Could you check a few things on this model? Use its own coordinates, in mm. Give positions to 0.01 mm unless a question says otherwise; leave off trailing zeros. Answer in a Markdown table with one row per item.
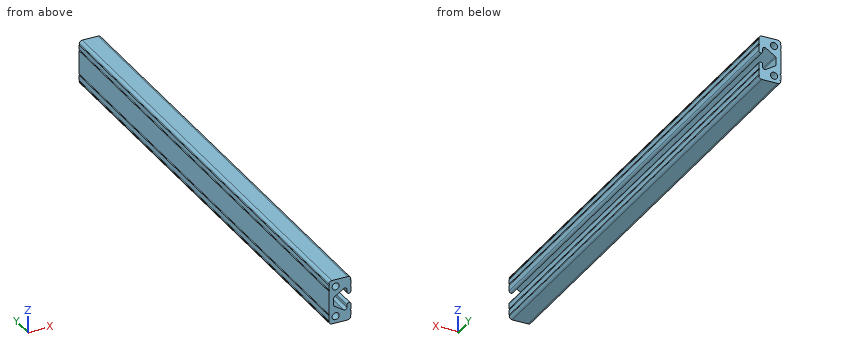
Solid Edge part; units mm, degrees
sketch "Sketch1" plane through (0, 0, 0) normal (0, 0, 1) x (1, 0, 0)
  line L0 (0, 0) -> (0, 279.4)
sketch "Sketch2" plane through (0, 0, 0) normal (0, -1, 0) x (1, 0, 0)
  line L0 (4.572, 12.7) -> (-4.572, 12.7)
  arc A0 (-4.572, 12.7) -> (-6.35, 10.922) centre (-4.572, 10.922) ccw
  line L1 (-6.35, 10.922) -> (-6.35, -10.922)
  arc A1 (-4.572, -12.7) -> (-6.35, -10.922) centre (-4.572, -10.922) cw
  line L2 (-4.572, -12.7) -> (4.572, -12.7)
  arc A2 (4.572, -12.7) -> (6.35, -10.922) centre (4.572, -10.922) ccw
  line L3 (6.35, -10.922) -> (6.35, 10.922)
  arc A3 (6.35, 10.922) -> (4.572, 12.7) centre (4.572, 10.922) ccw
sweep "SweptProtrusion1" add profiles "Sketch2" path "Sketch1"
sketch "Sketch3" plane through (0, 0, 0) normal (0, 0, 1) x (1, 0, 0)
  line L0 (0, 0) -> (0, 279.4)
sketch "Sketch4" plane through (-6.35, 0, 6.35) normal (0, -1, 0) x (1, 0, 0)
  circle A0 centre (3.9624, 2.3876) radius 2.032
sweep "SweptCutout1" cut profiles "Sketch4" path "Sketch3"
sketch "Sketch5" plane through (0, 0, 0) normal (0, 0, 1) x (1, 0, 0)
  line L0 (0, 0) -> (0, 279.4)
sketch "Sketch6" plane through (-6.35, 0, 6.35) normal (0, -1, 0) x (1, 0, 0)
  circle A0 centre (3.9624, -15.0876) radius 2.032
sweep "SweptCutout2" cut profiles "Sketch6" path "Sketch5"
sketch "Sketch7" plane through (0, 0, 0) normal (0, 0, 1) x (1, 0, 0)
  line L0 (0, 0) -> (0, 279.4)
sketch "Sketch8" plane through (0, 0, 0) normal (0, -1, 0) x (1, 0, 0)
  line L0 (4.1402, 3.7973) -> (4.1402, 5.2661)
  arc A0 (4.1402, 5.2661) -> (2.2806, 6.2777) centre (2.9353, 5.2661) ccw
  line L1 (-3.147, 2.7652) -> (2.2806, 6.2777)
  arc A1 (-3.495, 2.1255) -> (-3.147, 2.7652) centre (-2.733, 2.1255) cw
  line L2 (-3.495, 2.1255) -> (-3.495, -2.1255)
  arc A2 (-3.495, -2.1255) -> (-3.147, -2.7652) centre (-2.733, -2.1255) ccw
  line L3 (-3.147, -2.7652) -> (2.2806, -6.2777)
  arc A3 (4.1402, -5.2661) -> (2.2806, -6.2777) centre (2.9353, -5.2661) cw
  line L4 (4.1402, -3.7846) -> (4.1402, -5.2661)
  line L5 (6.35, 3.7973) -> (6.35, -3.7846)
  arc A4 (4.1402, -3.7846) -> (6.35, -3.7846) centre (5.2451, -3.7846) cw
  arc A5 (6.35, 3.7973) -> (4.1402, 3.7973) centre (5.2451, 3.7973) cw
sweep "SweptCutout3" cut profiles "Sketch8" path "Sketch7"
sketch "Sketch9" plane through (0, 0, 0) normal (0, 0, 1) x (1, 0, 0)
  line L0 (0, 0) -> (0, 279.4)
sketch "Sketch10" plane through (0, 0, 0) normal (0, -1, 0) x (-1, 0, 0)
  circle A0 centre (6.35, -10.795) radius 0.381
sweep "SweptCutout4" cut profiles "Sketch10" path "Sketch9"
sketch "Sketch11" plane through (0, 0, 0) normal (0, 0, 1) x (1, 0, 0)
  line L0 (0, 0) -> (0, 279.4)
sketch "Sketch12" plane through (0, 0, 0) normal (0, -1, 0) x (0, 0, 1)
  circle A0 centre (7.366, 6.35) radius 0.381
sweep "SweptCutout5" cut profiles "Sketch12" path "Sketch11"
sketch "Sketch13" plane through (0, 0, 0) normal (0, 0, 1) x (1, 0, 0)
  line L0 (0, 0) -> (0, 279.4)
sketch "Sketch14" plane through (0, 0, 0) normal (0, -1, 0) x (-1, 0, 0)
  circle A0 centre (-6.35, -10.795) radius 0.381
sweep "SweptCutout6" cut profiles "Sketch14" path "Sketch13"
sketch "Sketch15" plane through (0, 0, 0) normal (0, 0, 1) x (1, 0, 0)
  line L0 (0, 0) -> (0, 279.4)
sketch "Sketch16" plane through (0, 0, 0) normal (0, -1, 0) x (0, 0, 1)
  circle A0 centre (7.3678, -6.35) radius 0.381
sweep "SweptCutout7" cut profiles "Sketch16" path "Sketch15"
sketch "Sketch17" plane through (0, 0, 0) normal (0, 0, 1) x (1, 0, 0)
  line L0 (0, 0) -> (0, 279.4)
sketch "Sketch18" plane through (0, 0, 0) normal (0, -1, 0) x (0, 0, -1)
  circle A0 centre (10.795, -6.35) radius 0.381
sweep "SweptCutout8" cut profiles "Sketch18" path "Sketch17"
sketch "Sketch19" plane through (0, 0, 0) normal (0, 0, 1) x (1, 0, 0)
  line L0 (0, 0) -> (0, 279.4)
sketch "Sketch20" plane through (0.0001, 0, 0) normal (0, -1, 0) x (0, 0, -1)
  circle A0 centre (6.985, -6.3501) radius 0.381
sweep "SweptCutout9" cut profiles "Sketch20" path "Sketch19"
sketch "Sketch21" plane through (0, 0, 0) normal (0, 0, 1) x (1, 0, 0)
  line L0 (0, 0) -> (0, 279.4)
sketch "Sketch22" plane through (0.0001, 0, 0) normal (0, -1, 0) x (0, 0, -1)
  circle A0 centre (10.795, 6.3499) radius 0.381
sweep "SweptCutout10" cut profiles "Sketch22" path "Sketch21"
sketch "Sketch23" plane through (0, 0, 0) normal (0, 0, 1) x (1, 0, 0)
  line L0 (0, 0) -> (0, 279.4)
sketch "Sketch24" plane through (0.0001, 0, 0) normal (0, -1, 0) x (0, 0, 1)
  circle A0 centre (-7.0993, -6.3499) radius 0.3937
sweep "SweptCutout11" cut profiles "Sketch24" path "Sketch23"
1) Will these pins go through, and if not, where does the flat tip stop? P1, Ø1.3, axis at y = 172, z = 0.5, coming from the +X side (3 decimals); P2, Ø4, axis at y = 138.5, z = 1.5, coming from the +X side.
Check values:
| item | result |
|---|---|
| P1 | stops at x = -3.495 |
| P2 | stops at x = 6.31 |
2) If I drill on line 1 (X direction, y = 216, z = 8.75); line 2 (Z direction, x = -3.25, y = 39); line 3 (Z direction, x = 2.75, y = 163.5), over which ranges is the centre line in solid material (lowest first)?
Check values:
| item | result |
|---|---|
| line 1 | x = -6.35 to -4.42, -0.36 to 6.35 |
| line 2 | z = -12.7 to -10.58, -6.9 to -2.69, 2.69 to 6.9, 10.58 to 12.7 |
| line 3 | z = -12.7 to -6.46, 6.46 to 12.7 |
3) Imagine slicing it at A-A (y = 33.5). State how many separate pieces and enclosed holes the cut face has, then the cut area to 3 significant figures.
Check values:
| item | result |
|---|---|
| separate pieces | 1 |
| enclosed holes | 2 |
| area | 205 mm2 |
